Could you check a few things on this drawing? It's one solid part, dimensions in mm from its lowest x, y, z. A direction names the side the tool comes from. Give positions to 0.01 mm unless a question says otherwise; leave off trailing zeros. Order: outer loops, then holes, each group sorted by start corner. A loop starts at its lowest first (then second) coordinate and runs counter-clockwise, first axis right, second up.
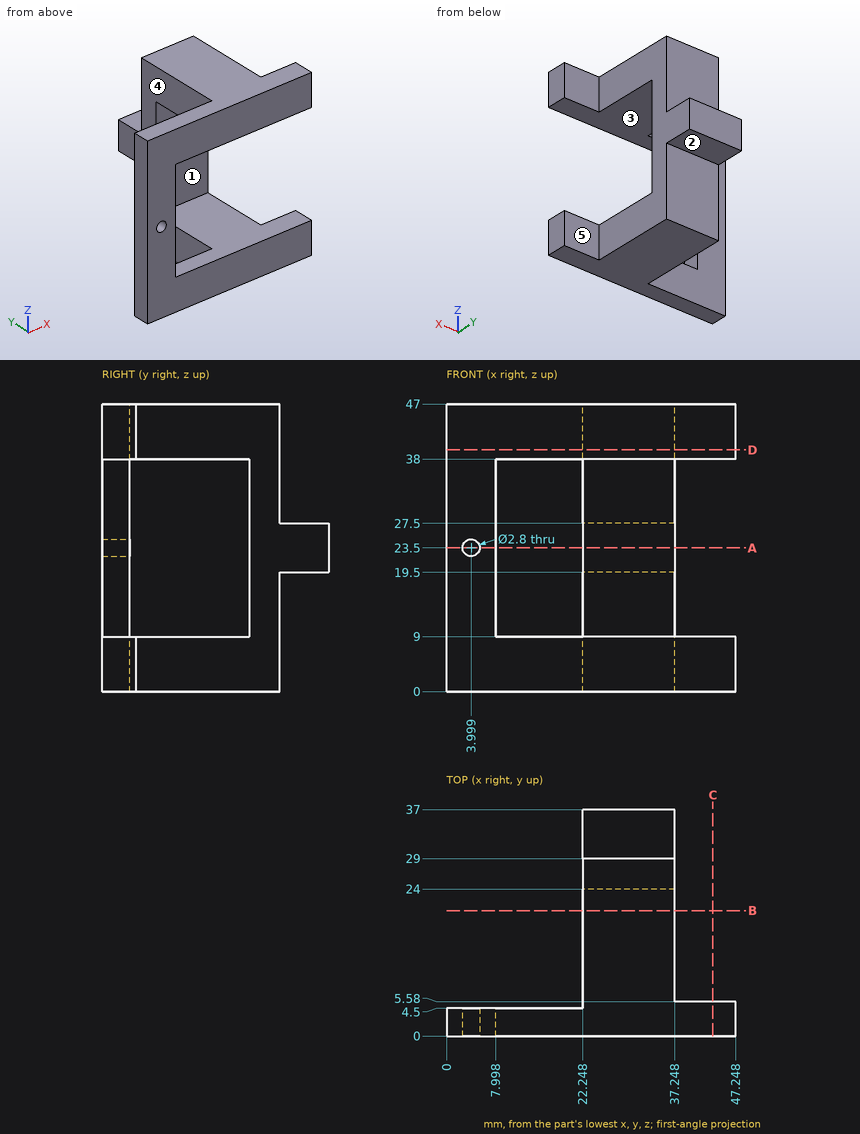
Q1. For the marked faces 1, 2, 3, 4 and 5, which set-ups out of +Z, -Z, +X, -X, +Y, -Y let a thin tool reach every point of the face, with its end or its side?
Filled sheet:
face 1: +X, -X, -Y
face 2: -Z, +X, -X, +Y
face 3: +X, -Y
face 4: +Z, -Z, -X, +Y
face 5: +Z, -Z, +X, +Y
Q2. If we section it at D-D on z = 39.5: List the corners of the cut face in (x, y) for me.
Filled sheet:
outline: (0, 0) - (47.25, 0) - (47.25, 5.58) - (37.25, 5.58) - (37.25, 29) - (22.25, 29) - (22.25, 4.5) - (0, 4.5) - close
Q3. I need wall thicknesses on L1, parallel to Z at x = 25, y = 8.5; L2, parallel to X at y = 3.05, z = 23.5; L3, parallel to Y at x = 3.5, z = 30. Which ranges of each line are inside material? Lowest first, please.
Filled sheet:
L1: z = 0 to 9, 38 to 47
L2: x = 0 to 2.6, 5.4 to 8
L3: y = 0 to 4.5
Q4. I'm going to push flat-ended pins straight in: P1, Ø12, axis at y = 23.5, z = 15, coming from the -X side; P2, Ø12, axis at x = 27, z = 35, coming from the +Y side; P3, Ø7.5, axis at x = 32.5, z = 29, coming from the -Y side; P4, Ø7, axis at x = 18.5, y = 16, coming from the -Z side. Where does each tip first touch, or does it pass through?
Filled sheet:
P1: stops at x = 22.25
P2: stops at y = 29
P3: stops at y = 24
P4: passes through
Q5. If we section it at B-B on y = 20.5: List the corners of the cut face in (x, z) for me, plus the area to 3 significant figures.
Filled sheet:
outline: (22.25, 0) - (37.25, 0) - (37.25, 9) - (22.25, 9) - close; (22.25, 38) - (37.25, 38) - (37.25, 47) - (22.25, 47) - close
area: 270 mm2
Q6. If we section it at C-C on x = 43.5: List the corners of the cut face in (y, z) for me, plus the area to 3 significant figures.
Filled sheet:
outline: (0, 0) - (5.58, 0) - (5.58, 9) - (0, 9) - close; (0, 38) - (5.58, 38) - (5.58, 47) - (0, 47) - close
area: 100 mm2
Q7. If we section it at A-A on z = 23.5: List the corners of the cut face in (x, y) for me.
Filled sheet:
outline: (0, 0) - (2.6, 0) - (2.6, 4.5) - (0, 4.5) - close; (5.4, 0) - (8, 0) - (8, 4.5) - (5.4, 4.5) - close; (22.25, 24) - (37.25, 24) - (37.25, 37) - (22.25, 37) - close
